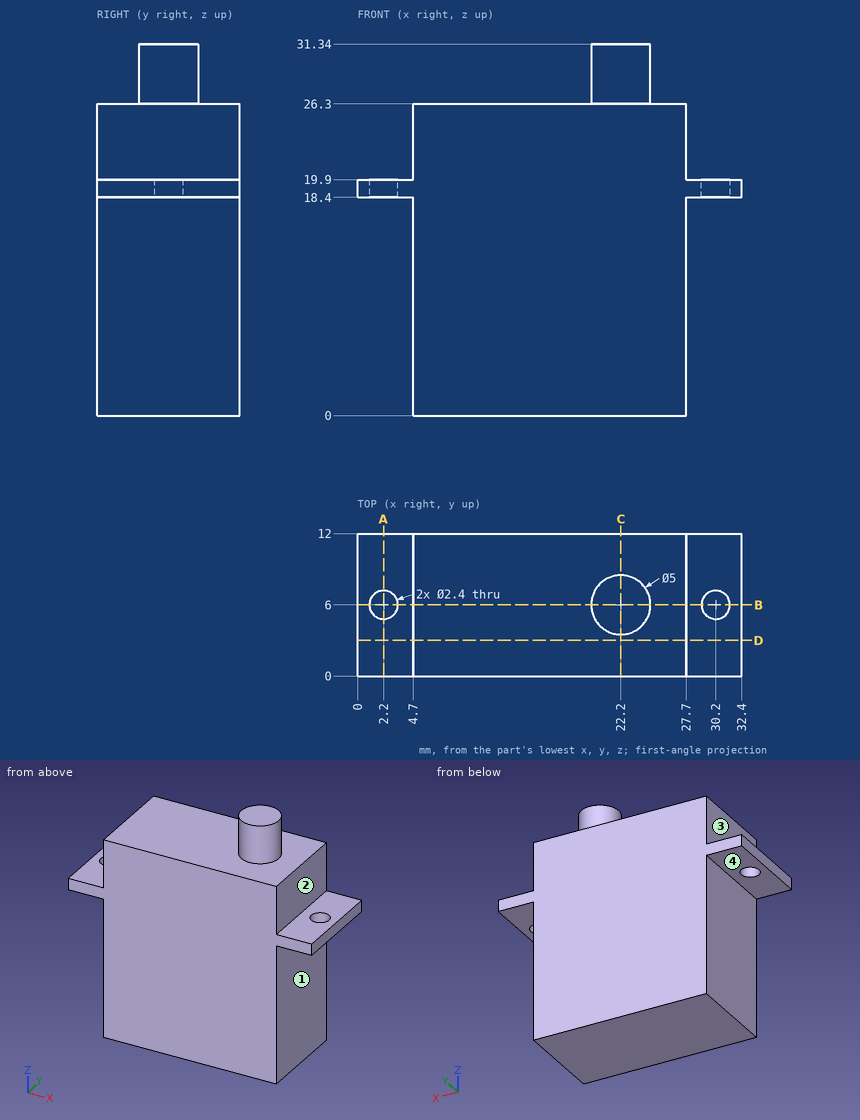
Print and shaded views of the part. All mm, measured from the part's lowest x, y and z. A direction names the side the tool comes from. Coordinates: 2 decimals unless noted, no trailing zeros. Order: outer loops, then holes, each group sorted by start corner. A loop starts at its lowest first (then second) coordinate and runs counter-clockwise, first axis right, second up. Notation, with made-up numbers: (71, 11) -> (87, 11) arc R4 cw to (87, 18) -> close; hole circle Ø3 at (69, -23.5). An arc over 180 degrees is marked (long way). Answer as a JSON object with one key per item and string values. Group by question number.
1) Cut at A-A, the plane x = 2.2. Write the cut outline in (y, z).
2) Cut at C-C, the plane x = 22.2. Write the cut outline in (y, z), then the cut area to 3 significant figures.
3) Which spindle directions (+Z, -Z, +X, -X, +Y, -Y) get a long thin tool onto all of the face, cutting with end or side? Do the marked faces 1, 2, 3 and 4. Say none if no direction does.
4) Cut at B-B, the plane y = 6. Write the cut outline in (x, z), then the cut area to 3 significant figures.
5) Cut at D-D, the plane y = 3. Write the cut outline in (x, z).
6) Flat gauge pins, fed straight in: pin 1 (2.5 mm diameter, centred on x = 30, y = 6.5, fed in from +Z); pin 2 (6 mm diameter, centred on y = 7.5, z = 14.5, fed in from +X); pin 3 (4 mm diameter, centred on x = 4.5, z = 26.5, fed in from -Y); pin 4 (2 mm diameter, centred on y = 6.5, z = 6.5, fed in from -X). Where does each tip first touch, or does it go through?
7) Drill centre lines: L1, parallel to Y at x = 2.2, z = 19.1; L2, parallel to X at y = 4.25, z = 23; L3, parallel to Z at x = 17.5, y = 4.75. Where is each one in solid material? Low to high.
Check values:
{
 "1": {"outline": "(0, 18.4) -> (4.8, 18.4) -> (4.8, 19.9) -> (0, 19.9) -> close; (7.2, 18.4) -> (12, 18.4) -> (12, 19.9) -> (7.2, 19.9) -> close"},
 "2": {"outline": "(0, 0) -> (12, 0) -> (12, 26.3) -> (8.5, 26.3) -> (8.5, 31.34) -> (3.5, 31.34) -> (3.5, 26.3) -> (0, 26.3) -> close", "area": "341 mm²"},
 "3": {"face 1": "-Z, +X, +Y, -Y", "face 2": "+Z, +X, +Y, -Y", "face 3": "+Z, -X, +Y, -Y", "face 4": "-Z, -X, +Y, -Y"},
 "4": {"outline": "(0, 18.4) -> (1, 18.4) -> (1, 19.9) -> (0, 19.9) -> close; (3.4, 18.4) -> (4.7, 18.4) -> (4.7, 0) -> (27.7, 0) -> (27.7, 18.4) -> (29, 18.4) -> (29, 19.9) -> (27.7, 19.9) -> (27.7, 26.3) -> (24.7, 26.3) -> (24.7, 31.34) -> (19.7, 31.34) -> (19.7, 26.3) -> (4.7, 26.3) -> (4.7, 19.9) -> (3.4, 19.9) -> close; (31.4, 18.4) -> (32.4, 18.4) -> (32.4, 19.9) -> (31.4, 19.9) -> close", "area": "637 mm²"},
 "5": {"outline": "(0, 18.4) -> (4.7, 18.4) -> (4.7, 0) -> (27.7, 0) -> (27.7, 18.4) -> (32.4, 18.4) -> (32.4, 19.9) -> (27.7, 19.9) -> (27.7, 26.3) -> (4.7, 26.3) -> (4.7, 19.9) -> (0, 19.9) -> close"},
 "6": {"pin 1": "stops at z = 19.9", "pin 2": "stops at x = 27.7", "pin 3": "stops at y = 0", "pin 4": "stops at x = 4.7"},
 "7": {"L1": "y = 0 to 4.8, 7.2 to 12", "L2": "x = 4.7 to 27.7", "L3": "z = 0 to 26.3"}
}
